Could you check a few things on this model? Use its own coordinates, in mm. A direction names the side the tool comes from. Round coordinates to 2 decimals unless told otherwise and drop trailing zeros. Loops run counter-clockwise (first coordinate to the right, second up) from the corner with the lowest first, then second, coordinate; pieces in that order, holes last. Notation, with made-up numbers: (10.5, 30) - (45.5, 30) arc R12 ccw to (45.5, 44) - close; hole circle Ø4 at (-21.75, -1). An arc over 180 degrees is marked (long way). Use one line per item in the form item = value.
```python
from build123d import *

# Parameters (mm, degrees)
F0_W     = 42
F0_H     = 13
F0_R     = 1.75
F1_DEPTH = 8
F2_W     = 24
F2_H     = 6
F3_DEPTH = 2.5
F4_R     = 5.99999
F5_SIZE  = 3
F6_R     = 1.65
F6_R_2   = 2
F7_DEPTH = 13.001


# Not quite as in the source:
# - a fillet or chamfer is up to 0.001 mm smaller than in the source, because OpenCascade refuses the exact size


with BuildPart() as f1:
    # F0 (on Top) → F1 (new body, symmetric)
    with BuildSketch(Plane.XY):
        Rectangle(F0_W, F0_H)
        with Locations((-15.5, -1)):
            Circle(F0_R, mode=Mode.SUBTRACT)
        with Locations((15.5, -1)):
            Circle(F0_R, mode=Mode.SUBTRACT)
    extrude(amount=F1_DEPTH, both=True)

    # F2 (on face) → F3 (cut)
    with BuildSketch(Plane.XY.offset(8)):
        with Locations((0, 3.5)):
            Rectangle(F2_W, F2_H)
    extrude(amount=-F3_DEPTH, mode=Mode.SUBTRACT)

    # F4 (radius 6 in the source; OpenCascade refuses exactly that, so slightly less here)
    f4_edges = [f1.edges().sort_by_distance(p)[0] for p in [
        (-12, 0.5, 6.75),
        (12, 0.5, 6.75),
    ]]
    fillet(f4_edges, radius=F4_R)

    # F5
    f5_edges = [f1.edges().sort_by_distance(p)[0] for p in [
        (-21, -6.5, 0),
        (21, -6.5, 0),
    ]]
    chamfer(f5_edges, length=F5_SIZE)

    # F6 (on face) → F7 (cut, through all)
    with BuildSketch(Plane(origin=(0, 6.5, 0), x_dir=(-1, 0, 0), z_dir=(0, 1, 0))):
        with Locations((12, -2.5)):
            Circle(F6_R)
        with Locations((-6, -2.5)):
            Circle(F6_R_2)
    extrude(amount=-F7_DEPTH, mode=Mode.SUBTRACT)


solid = f1.part
```
1. If we section it at D-D, the plane z = -5: Write out the boundary of the cut face in (x, y), plus the area to 3 significant figures.
Solution:
outline = (-21, -3.5) - (-18, -6.5) - (18, -6.5) - (21, -3.5) - (21, 6.5) - (-21, 6.5) - close; hole circle Ø3.5 at (-15.5, -1); hole circle Ø3.5 at (15.5, -1)
area = 518 mm^2
2. We'd pull the mould along Y, two halves only. Please class faces 1 (the face through (0, 4, 5.5)), 2 (the face through (-10.289, 2.304, 6.732)), 3 (the face through (-13.831, -0.474, -0.112)): +Y half, -Y half, draft (parallel to the pull), parting line (faces both ways), or undercut.
Solution:
face_1 = draft
face_2 = +Y half
face_3 = undercut
3. If we section it at A-A, the plane y = -1: Write out the boundary of the cut face in (x, z), plus the area to 3 significant figures.
Solution:
outline = (-21, -8) - (-17.25, -8) - (-17.25, 8) - (-21, 8) - close; (-13.75, -8) - (13.75, -8) - (13.75, 8) - (-13.75, 8) - close; (17.25, -8) - (21, -8) - (21, 8) - (17.25, 8) - close; hole circle Ø3.3 at (-12, -2.5); hole circle Ø4 at (6, -2.5)
area = 539 mm^2
4. If we section it at B-B, the plane x = -15.5: Write out the boundary of the cut face in (y, z), plus the area to 3 significant figures.
Solution:
outline = (-6.5, -8) - (-2.75, -8) - (-2.75, 8) - (-6.5, 8) - close; (0.75, -8) - (6.5, -8) - (6.5, 8) - (0.75, 8) - close
area = 152 mm^2
5. Please list where these lines run through material, in increasing order: line 1 along X through (y, z) = (-1.5, -0.75); line 2 along Z through (x, y) = (6, -0.75); line 3 along Y through (x, z) = (-15.5, -0.75).
Solution:
line_1 = -21 to -17.18, -13.82 to 5.03, 6.97 to 13.82, 17.18 to 21
line_2 = -8 to -4.5, -0.5 to 8
line_3 = -6.5 to -2.75, 0.75 to 6.5
6. If we section it at C-C, the plane z = -2.5: Write out the boundary of the cut face in (x, y), plus the area to 3 significant figures.
Solution:
outline = (-21, -3.5) - (-18, -6.5) - (-13.65, -6.5) - (-13.65, 6.5) - (-21, 6.5) - close; (-10.35, -6.5) - (4, -6.5) - (4, 6.5) - (-10.35, 6.5) - close; (8, -6.5) - (18, -6.5) - (21, -3.5) - (21, 6.5) - (8, 6.5) - close; hole circle Ø3.5 at (-15.5, -1); hole circle Ø3.5 at (15.5, -1)
area = 423 mm^2
7. For P1, Ø1.2, axis at x = 0.5, z = 7, coming from the +Y side; P2, Ø3, axis at x = -3, y = 4.5, coming from the +Z side, each with a flat end and sliding along its axis, tell me the tip position at first contact or that it passes through.
Solution:
P1 = 0.5
P2 = 5.5
8. On a 3-axis mill with a long thin cutter (end or side, diameter ignored), from which of +Z, -Z, +X, -X, +Y, -Y can I reach the whole of each face in a straight line? I mean faces 4 (the face through (0, -1, 8)), 5 (the face through (10.289, 2.304, 6.732)). Say none if no direction works.
Solution:
face_4 = +Z, +X, -X, +Y, -Y
face_5 = +Z, +Y
